CAD build for the part. Positions are in the model's coordinates, mm. Round coordinates to 2 decimals unless told otherwise and drop trailing zeros. Write each loop counter-clockwise with the first axis right and the second up, starting at its lowest first coordinate (ties: lowest second). Pieces come first, ordered by that corner, then holes. Notation, with made-up numbers: (23.25, -30) - (52.25, -30) arc R25 ccw to (52.25, -12) - close; hole circle Ø4 at (16, 0). An arc over 180 degrees is marked (long way). Put each result on its own line as item: value. Start each with the question number.
Item 1: Cut at A-A (z = 80). Give the cut face in (x, y), and give its area (3 significant figures).
Item 2: Drill centre lines: line 1 (X direction, y = -18, z = -21); line 2 (X direction, y = 29, z = -12); line 3 (Y direction, x = -20, z = 50). Where is each one in solid material? Low to high. Write a range as from..to.
Item 3: Cut at B-B (z = 0). Give the cut face in (x, y).
Item 4: Pin check, flat tips, straight feed: pin 1 Ø4 at (x, z) = (-17, 30) entering from +Y; pin 2 Ø10 at (x, z) = (4.5, -7.5) entering from +Y; pin 3 Ø8 at (x, z) = (-34, -25) entering from +Y. Stop position of each tip, or through.
Item 5: Mould opens along Y. For faces 1 (the conical face through (-0.23, 0.18, 101.19)), 2 (the flat face through (-52, 12, -49.924)), 3 (the conical face through (23.87, 9.9, 41.15)) say: released by +Y, released by -Y, zero draft, split by the parting line, or undercut.
```python
from build123d import *

# Parameters (mm, degrees)
F2_T = -1.27
F3_R = 7.0358


with BuildPart() as f1:
    # F0 (on Front) → F1 (revolve)
    with BuildSketch(Plane.XZ):
        Polygon((0, 102.476016), (0, -49.923984), (53.975, -49.923984), (7.011191, 102.107614), align=None)
    revolve(axis=Axis((0, 0, 26.276016), (0, 0, -1)))

    # F2
    f2_openings = [f1.faces().sort_by_distance(p)[0] for p in [
        (0, 0, -49.923984),
    ]]
    offset(amount=F2_T, openings=f2_openings)

    # F3
    f3_edges = [f1.edges().sort_by_distance(p)[0] for p in [
        (-7.011191, 0, 102.107614),
    ]]
    fillet(f3_edges, radius=F3_R)


solid = f1.part
```
Output values:
1. outline: circle Ø27.68 at (0, 0); hole circle Ø25.02 at (0, 0)
1. area: 110 mm2
2. line 1: -41.29..-39.83, 39.83..41.29
2. line 2: -30.74..-28.88, 28.88..30.74
2. line 3: -11.57..-8.62, 8.62..11.57
3. outline: circle Ø77.11 at (0, 0); hole circle Ø74.45 at (0, 0)
4. pin 1: y = 25.35
4. pin 2: y = 42.24
4. pin 3: y = 35.6
5. face 1: undercut
5. face 2: zero draft
5. face 3: split by the parting line
